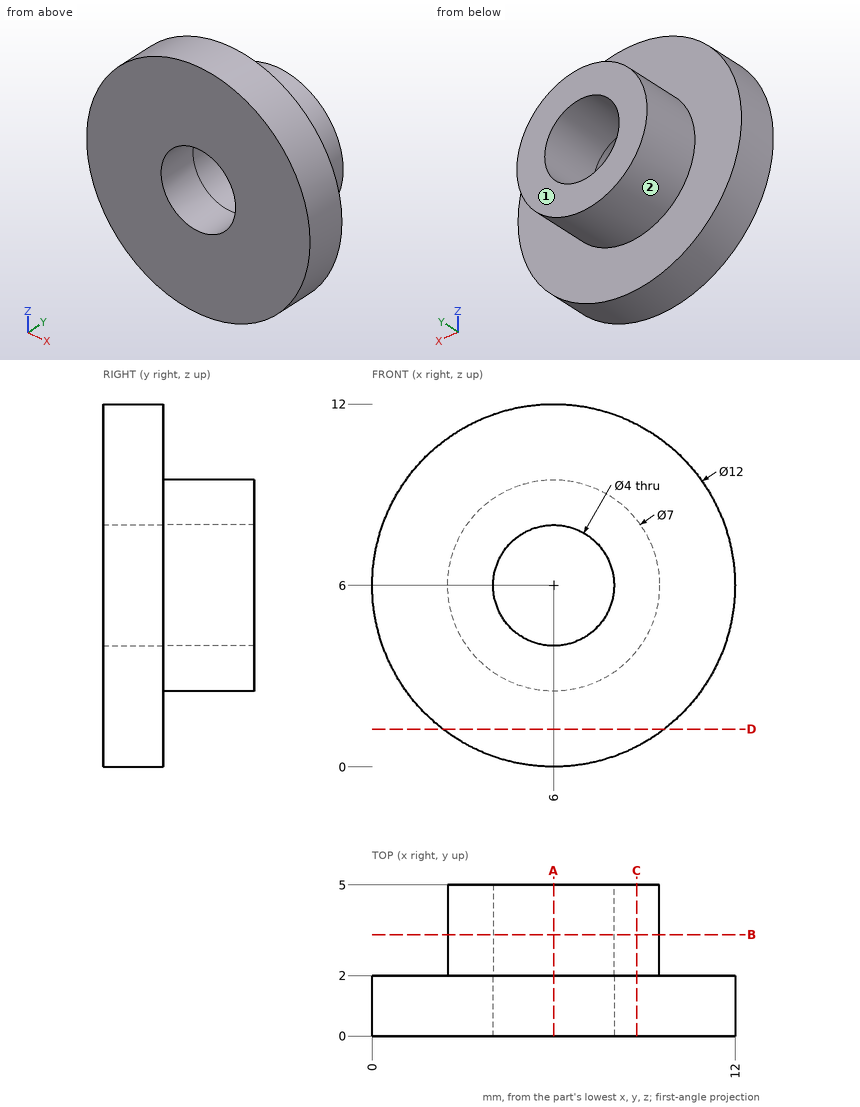
Job drawing, mm, ordinate dimensions from the low corner. One solid piece. A direction names the side the tool comes from. Give positions to 0.01 mm unless a question says otherwise; leave off trailing zeros. Loops run counter-clockwise (first coordinate to the right, second up) from the corner with the lowest first, then second, coordinate; pieces in that order, holes last. Notation, with made-up numbers: (86.5, 78.5) -> (133.5, 78.5) arc R26 cw to (133.5, 115.5) -> close; hole circle Ø11 at (80, 58.5). An arc over 180 degrees is marked (long way). Write each question's results on one line, items separated by ' | '.
(1) Tool access for the marked faces 1 and 2: list every direction of +Z, -Z, +X, -X, +Y, -Y with a clear straight run to the whole face (end or side of a thin tool).
Geometry results:
face 1: +Z, -Z, +X, -X, +Y | face 2: +Y
(2) Cut at A-A on x = 6. List the corners of the cut face in (y, z), and give its area (3 significant figures).
Geometry results:
outline: (0, 0) -> (2, 0) -> (2, 2.5) -> (5, 2.5) -> (5, 4) -> (0, 4) -> close; (0, 8) -> (5, 8) -> (5, 9.5) -> (2, 9.5) -> (2, 12) -> (0, 12) -> close | area: 25.0 mm²
(3) Cut at C-C on x = 8.75. List the corners of the cut face in (y, z), and give its area (3 significant figures).
Geometry results:
outline: (0, 0.67) -> (2, 0.67) -> (2, 3.83) -> (5, 3.83) -> (5, 8.17) -> (2, 8.17) -> (2, 11.33) -> (0, 11.33) -> close | area: 34.3 mm²
(4) Cut at B-B on y = 3.35. List the corners of the cut face in (x, z).
Geometry results:
outline: circle Ø7 at (6, 6); hole circle Ø4 at (6, 6)
(5) Flat gauge pins, fed straight in: pin 1 Ø2 at (x, y) = (5, 3.5) entering from -Z; pin 2 Ø1.5 at (y, z) = (4, 1.5) entering from +X; pin 3 Ø1.5 at (x, y) = (2.5, 3) entering from +Z. Where does each tip first touch, or does it go through?
Geometry results:
pin 1: stops at z = 2.5 | pin 2: passes through | pin 3: stops at z = 8.17
(6) Probe line 1 along Z through (x, y) = (6, 2.65); line 2 along X through (y, z) = (0.95, 6). List the from-to ranges inside material, lowest first.
Geometry results:
line 1: z = 2.5 to 4, 8 to 9.5 | line 2: x = 0 to 4, 8 to 12
(7) Cut at D-D on z = 1.25. List the corners of the cut face in (x, y).
Geometry results:
outline: (2.33, 0) -> (9.67, 0) -> (9.67, 2) -> (2.33, 2) -> close
